Part model, mm, in its own coordinate system. A direction names the side the tool comes from. Give positions to 0.01 mm unless a question says otherwise; leave off trailing zeros. Order: outer loops, then holes, each group sorted by start corner. A loop starts at its lowest first (then second) coordinate and runs counter-clockwise, first axis right, second up. Notation, with made-up numbers: M 36,-21 L 78,-21 A19 ccw 78,0 Z; hole C 72.25,61.25 d3. An arc over 180 degrees is marked long. Answer as a JSON object with one key per item and string values.
from build123d import *

# Parameters (mm, degrees)
F1_DEPTH  = 11
F3_W      = 3
F3_H      = 20
F3_W_2    = 3.4
F3_H_2    = 10.2
F4_DEPTH  = 25
F5_R      = 1.5
F6_DEPTH  = 25
F5_R_2    = 2.5
F7_DEPTH  = 8
F8_SIZE   = 1.49999
F9_SIZE   = 1.49999
F10_R     = 7.5
F12_DEPTH = 0.5


# Not quite as in the source:
# - a fillet or chamfer is up to 0.001 mm smaller than in the source, because OpenCascade refuses the exact size


with BuildPart() as f1:
    # F0 (on Front) → F1 (new body)
    with BuildSketch(Plane.XZ):
        Polygon((-4, 0), (0, 0), (0, 9.8), (-1.7, 9.8), (-1.7, 22.5), (-4, 22.5), align=None)
    extrude(amount=F1_DEPTH)

    # F2: F1 across face


with BuildPart() as f1_1:
    add(f1.part)
    add(f1.part.mirror(Plane(origin=(0, -5.5, 4.9), x_dir=(0, 1, 0), z_dir=(1, 0, 0))))

    # F3 (on face) → F4 (join)
    with BuildSketch(Plane.XZ.offset(11)):
        with Locations((5.5, 10)):
            Rectangle(F3_W, F3_H)
        with Locations((0, 14.9)):
            Rectangle(F3_W_2, F3_H_2)
        Polygon((-4, 0), (0, 0), (4, 0), (4, 20), (1.7, 20), (1.7, 9.8), (-1.7, 9.8), (-1.7, 20), (-4, 20), align=None)
        with Locations((-5.5, 10)):
            Rectangle(F3_W, F3_H)
    extrude(amount=F4_DEPTH)

    # F5 (on face) → F6 (cut)
    with BuildSketch(Plane.YZ.offset(4)):
        with Locations((-4, 16)):
            Circle(F5_R)
    extrude(amount=-F6_DEPTH, mode=Mode.SUBTRACT)

    # F5 (on face) → F7 (join, through all)
    with BuildSketch(Plane.YZ.offset(4)):
        with Locations((-4, 16)):
            Circle(F5_R_2)
        with Locations((-4, 16)):
            Circle(F5_R, mode=Mode.SUBTRACT)
    extrude(amount=-F7_DEPTH)

    # F8 (size 1.5 in the source; OpenCascade refuses exactly that, so slightly less here)
    f8_edges = [f1_1.edges().sort_by_distance(p)[0] for p in [
        (-1.7, -6.5, 16),
    ]]
    chamfer(f8_edges, length=F8_SIZE)

    # F9 (size 1.5 in the source; OpenCascade refuses exactly that, so slightly less here)
    f9_edges = [f1_1.edges().sort_by_distance(p)[0] for p in [
        (1.7, -6.5, 16),
    ]]
    chamfer(f9_edges, length=F9_SIZE)

    # F10 (on face) → F12 (join)
    with BuildSketch(Plane(origin=(0, 0, 0), x_dir=(-1, 0, 0), z_dir=(0, 1, 0))):
        with Locations((0, 16.6603474262)):
            Circle(F10_R)
    extrude(amount=F12_DEPTH)


solid = f1_1.part
1. Probe line 1 along Y through (x, z) = (-6.75, 18.75); line 2 along Z through (x, y) = (-1.25, -4); line 3 along Z through (x, y) = (-1.5, -4). List the from-to ranges inside material, lowest first.
Worked answers:
{"line 1": "y = -36 to -11, 0 to 0.5", "line 2": "z = 0 to 9.8, 12.45 to 14.5, 17.5 to 19.55", "line 3": "z = 0 to 9.8, 12.2 to 14.5, 17.5 to 19.8"}
2. Two-plate mould, pull along X, no slides. Class faces 5 (the flat face through (0, -11, 15)), 6 (the flat face through (0, 0.5, 17)), 7 (the flat face through (4, -5, 11)): +X half, -X half, draft (parallel to the pull), parting line (faces both ways), or undercut.
Worked answers:
{"face 5": "undercut", "face 6": "draft", "face 7": "+X half"}
3. Cut at B-B on x = -1.25. Give the cut face in (y, z), plus the area to 3 significant figures.
Worked answers:
{"outline": "M -36,0 L 0,0 L 0,9.27 L 0.5,9.27 L 0.5,24.06 L 0,24.06 L 0,9.8 L -11,9.8 L -11,20 L -36,20 Z; C -4,16 d7.1; hole C -4,16 d3", "area": "648 mm^2"}
4. Cut at D-D on x = 4.5. Give the cut face in (y, z).
Worked answers:
{"outline": "M -36,0 L -11,0 L -11,20 L -36,20 Z; M 0,10.66 L 0.5,10.66 L 0.5,22.66 L 0,22.66 Z"}
5. Cut at C-C on z = 8. Give the cut face in (x, y).
Worked answers:
{"outline": "M -7,-36 L 7,-36 L 7,-11 L 4,-11 L 4,0 L -4,0 L -4,-11 L -7,-11 Z"}
6. Which spindle directions (+Z, -Z, +X, -X, +Y, -Y) get a long thin tool onto all of the face, cutting with end or side? Do faces 1 (the flat face through (5, -11, 10)), 2 (the flat face through (0, 0, 17)), 3 (the flat face through (-3, -11, 21)), 4 (the flat face through (0, -5, 9.8)). Say none if no direction does.
Worked answers:
{"face 1": "+Z, -Z, +X", "face 2": "+Z", "face 3": "+Z, +X, -X, -Y", "face 4": "none"}
7. Cut at A-A on y = -4. Give the cut face in (x, z), plus the area to 3 significant figures.
Worked answers:
{"outline": "M -4,0 L 4,0 L 4,14.5 L -4,14.5 Z; M -4,17.5 L 4,17.5 L 4,22.5 L 1.7,22.5 L 1.7,20 L 0.2,18.5 L -0.2,18.5 L -1.7,20 L -1.7,22.5 L -4,22.5 Z; hole M -1.7,9.8 L 1.7,9.8 L 1.7,12 L 0.2,13.5 L -0.2,13.5 L -1.7,12 Z", "area": "134 mm^2"}
8. Pin check, flat tips, straight feed: P1, Ø2.5, axis at x = 5.5, z = 7.5, coming from the +Y side; P2, Ø8, axis at y = -11.5, z = 8.5, coming from the +X side; P3, Ø1.8, axis at x = -2.5, y = -7.5, coming from the +Z side. Stop position of each tip, or through.
Worked answers:
{"P1": "stops at y = -11", "P2": "stops at x = 7", "P3": "stops at z = 22.5"}
